Print and shaded views of the part. All mm, measured from the part's lowest x, y and z. A direction names the side the tool comes from. Round coordinates to 2 decimals unless told otherwise and drop trailing zeros. Order: outer loops, then holes, each group sorted by start corner. A loop starts at its lowest first (then second) coordinate and runs counter-clockwise, first axis right, second up. Notation, with made-up numbers: (75, 52.25) - (123, 52.25) arc R11 cw to (123, 59.25) - close; hole circle Ø2 at (62, 8.25). An arc over 180 degrees is marked (long way). Write item = value, one per line.
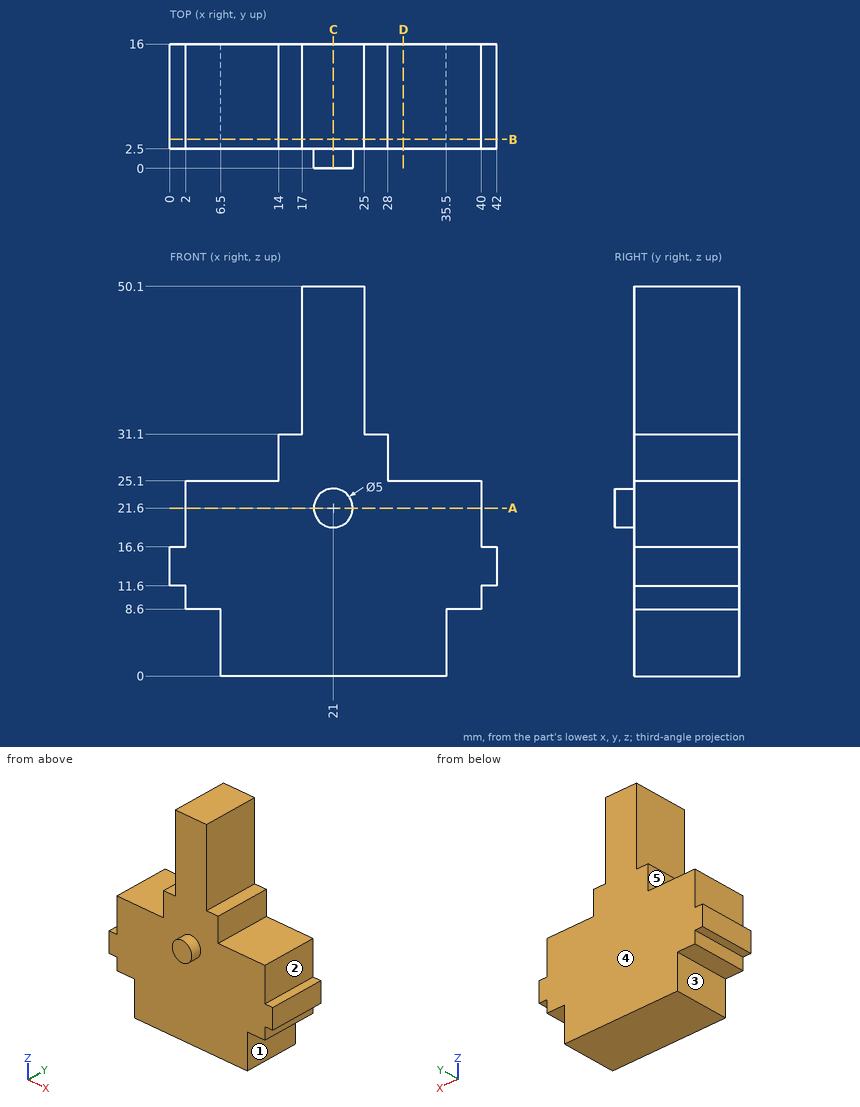
(1) Probe line 1 along Z through (x, y) = (4.5, 11); line 2 along Z through (x, y) = (26.5, 13.25); line 3 along Y through (x, z) = (20, 4). List the from-to ranges inside material, lowest first.
Solved:
line_1 = 8.6 to 25.1
line_2 = 0 to 31.1
line_3 = 2.5 to 16
(2) Tool access for the marked faces 1, 2, 3, 4 and 5: list every direction of +Z, -Z, +X, -X, +Y, -Y with a clear straight run to the whole face (end or side of a thin tool).
Solved:
face_1 = -Z, +X, +Y, -Y
face_2 = +Z, +X, +Y, -Y
face_3 = -Z, -X, +Y, -Y
face_4 = +Z, -Z, +X, -X, +Y
face_5 = +Z, -X, +Y, -Y
(3) Band-saw the part on A-A on z = 21.6. List the corners of the cut face in (x, y), plus the area to 4 significant figures.
Solved:
outline = (2, 2.5) - (18.5, 2.5) - (18.5, 0) - (23.5, 0) - (23.5, 2.5) - (40, 2.5) - (40, 16) - (2, 16) - close
area = 525.5 mm²
(4) Band-saw the part on B-B on y = 3.75. List the corners of the cut face in (x, z), plus the area to 3 significant figures.
Solved:
outline = (0, 11.6) - (2, 11.6) - (2, 8.6) - (6.5, 8.6) - (6.5, 0) - (35.5, 0) - (35.5, 8.6) - (40, 8.6) - (40, 11.6) - (42, 11.6) - (42, 16.6) - (40, 16.6) - (40, 25.1) - (28, 25.1) - (28, 31.1) - (25, 31.1) - (25, 50.1) - (17, 50.1) - (17, 31.1) - (14, 31.1) - (14, 25.1) - (2, 25.1) - (2, 16.6) - (0, 16.6) - close
area = 1,130 mm²
(5) Band-saw the part on D-D on x = 30. List the corners of the cut face in (y, z).
Solved:
outline = (2.5, 0) - (16, 0) - (16, 25.1) - (2.5, 25.1) - close
(6) Drop flat-ended pins along their axis: pin 1 (2.5 mm diameter, centred on y = 11.5, z = 20, fed in from -X); pin 2 (1.5 mm diameter, centred on x = 32, y = 9, fed in from +Z); pin 3 (1.5 mm diameter, centred on y = 10, z = 33, fed in from +X). Give the stop position or say it passes through.
Solved:
pin_1 = 2
pin_2 = 25.1
pin_3 = 25
(7) Band-saw the part on C-C on x = 21. List the corners of the cut face in (y, z).
Solved:
outline = (0, 19.1) - (2.5, 19.1) - (2.5, 0) - (16, 0) - (16, 50.1) - (2.5, 50.1) - (2.5, 24.1) - (0, 24.1) - close
